```python
from build123d import *

# Parameters (mm, degrees)
SKETCH1_W           = 75
SKETCH1_H           = 90
BOSS_EXTRUDE1_DEPTH = 10
FILLET1_R           = 10
SKETCH3_W           = 75
SKETCH3_H           = 7.5
BOSS_EXTRUDE2_DEPTH = 60
FILLET2_R           = 7.5
SKETCH2_R           = 3
CUT_EXTRUDE1_DEPTH  = 10
CUT_EXTRUDE2_DEPTH  = 10
FILLET3_R           = 0.5
FILLET4_R           = 0.5


with BuildPart() as part:
    # Sketch1 → Boss-Extrude1 (new body)
    with BuildSketch(Plane.XY):
        Rectangle(SKETCH1_W, SKETCH1_H)
    extrude(amount=BOSS_EXTRUDE1_DEPTH)

    # Fillet1
    fillet1_edges = [part.edges().sort_by_distance(p)[0] for p in [
        (-37.5, 45, 5),
        (37.5, 45, 5),
    ]]
    fillet(fillet1_edges, radius=FILLET1_R)

    # Sketch3 → Boss-Extrude2 (add)
    with BuildSketch(Plane.XY.offset(10)):
        with Locations((0, -41.25)):
            Rectangle(SKETCH3_W, SKETCH3_H)
    extrude(amount=BOSS_EXTRUDE2_DEPTH)

    # Fillet2
    fillet2_edges = [part.edges().sort_by_distance(p)[0] for p in [
        (0, -37.5, 10),
    ]]
    fillet(fillet2_edges, radius=FILLET2_R)

    # Sketch2 → Cut-Extrude1 (cut)
    with BuildSketch(Plane.XY):
        with Locations(Location((23.999417703, 30, 0), (0, 0, 180))):
            Circle(SKETCH2_R)
        with Locations(Location((13.999417703, 30, 0), (0, 0, 180))):
            Circle(SKETCH2_R)
        with Locations(Location((3.999417703, 30, 0), (0, 0, 180))):
            Circle(SKETCH2_R)
        with Locations(Location((-6.000582297, 30, 0), (0, 0, 180))):
            Circle(SKETCH2_R)
        with Locations(Location((-16.000582297, 30, 0), (0, 0, 180))):
            Circle(SKETCH2_R)
        with Locations(Location((-26.000582297, 30, 0), (0, 0, 180))):
            Circle(SKETCH2_R)
        with Locations(Location((13.999417703, 15, 0), (0, 0, 180))):
            Circle(SKETCH2_R)
        with Locations(Location((3.999417703, 15, 0), (0, 0, 180))):
            Circle(SKETCH2_R)
        with Locations(Location((-6.000582297, 15, 0), (0, 0, 180))):
            Circle(SKETCH2_R)
        with Locations(Location((-16.000582297, 15, 0), (0, 0, 180))):
            Circle(SKETCH2_R)
        with Locations(Location((-26.000582297, 15, 0), (0, 0, 180))):
            Circle(SKETCH2_R)
        with Locations(Location((13.999417703, 0, 0), (0, 0, 180))):
            Circle(SKETCH2_R)
        with Locations(Location((3.999417703, 0, 0), (0, 0, 180))):
            Circle(SKETCH2_R)
        with Locations(Location((-6.000582297, 0, 0), (0, 0, 180))):
            Circle(SKETCH2_R)
        with Locations(Location((-16.000582297, 0, 0), (0, 0, 180))):
            Circle(SKETCH2_R)
        with Locations(Location((-26.000582297, 0, 0), (0, 0, 180))):
            Circle(SKETCH2_R)
        with Locations(Location((13.999417703, -15, 0), (0, 0, 180))):
            Circle(SKETCH2_R)
        with Locations(Location((3.999417703, -15, 0), (0, 0, 180))):
            Circle(SKETCH2_R)
        with Locations(Location((-6.000582297, -15, 0), (0, 0, 180))):
            Circle(SKETCH2_R)
        with Locations(Location((-16.000582297, -15, 0), (0, 0, 180))):
            Circle(SKETCH2_R)
        with Locations(Location((-26.000582297, -15, 0), (0, 0, 180))):
            Circle(SKETCH2_R)
        with Locations(Location((23.999417703, 15, 0), (0, 0, 180))):
            Circle(SKETCH2_R)
        with Locations(Location((23.999417703, 0, 0), (0, 0, 180))):
            Circle(SKETCH2_R)
        with Locations(Location((23.999417703, -15, 0), (0, 0, 180))):
            Circle(SKETCH2_R)
    extrude(amount=CUT_EXTRUDE1_DEPTH, mode=Mode.SUBTRACT)

    # Sketch4 → Cut-Extrude2 (cut)
    with BuildSketch(Plane(origin=(0, -37.5, 0), x_dir=(1, 0, 0), z_dir=(0, 1, 0))):
        with BuildLine():
            Line((-9.5, -26.25), (-9.5, -61.25))
            ThreePointArc((-9.5, -61.25), (-12.5, -64.25), (-15.5, -61.25))
            Line((-15.5, -61.25), (-15.5, -26.25))
            ThreePointArc((-15.5, -26.25), (-12.5, -23.25), (-9.5, -26.25))
        make_face()
        with BuildLine():
            Line((9.5, -26.25), (9.5, -61.25))
            ThreePointArc((9.5, -61.25), (12.5, -64.25), (15.5, -61.25))
            Line((15.5, -61.25), (15.5, -26.25))
            ThreePointArc((15.5, -26.25), (12.5, -23.25), (9.5, -26.25))
        make_face()
    extrude(amount=-CUT_EXTRUDE2_DEPTH, mode=Mode.SUBTRACT)

    # Fillet3
    fillet3_edges = [part.edges().sort_by_distance(p)[0] for p in [
        (0, -37.5, 70),
    ]]
    fillet(fillet3_edges, radius=FILLET3_R)

    # Fillet4
    fillet4_edges = [part.edges().sort_by_distance(p)[0] for p in [
        (0, 45, 10),
        (-37.5, 2.5, 10),
        (-34.571067812, 42.071067812, 10),
        (-37.5, -41.5, 70),
        (-37.5, -37.5, 43.5),
        (-37.5, -37.646446609, 69.853553391),
        (37.5, -37.5, 43.5),
        (37.5, -37.646446609, 69.853553391),
        (34.571067812, 42.071067812, 10),
        (37.5, -41.5, 70),
        (37.5, 2.5, 10),
        (-37.5, -35.303300859, 12.196699141),
        (37.5, -35.303300859, 12.196699141),
    ]]
    fillet(fillet4_edges, radius=FILLET4_R)


solid = part.part
```
Check sheet for the modelled part. Datum: model origin and axes. Units: mm. A direction names the side the tool comes from. Round coordinates to 2 decimals unless told otherwise and drop trailing zeros. Loops run counter-clockwise (first coordinate to the right, second up) from the corner with the lowest first, then second, coordinate; pieces in that order, holes last. Notation, with made-up numbers: (-2, -20) - (38, -20) arc R23 cw to (38, 6) - close; hole circle Ø1 at (43.25, 57). An arc over 180 degrees is marked (long way). Answer as a JSON object with one key per item and string values. Group by question number.
Q1. Sectioned sample at B-B, the plane x = 25. Enter the section's corners in (y, z), plus the area to 3 significant figures.
Q2. Scan lines: line 1 along Z through (x, y) = (-21.5, -20); line 2 along Y through (x, z) = (-16, 49); line 3 along Y through (x, z) = (-27.5, 4). Record each from-to range of solid material in increasing order. Write a range as [from, to].
Q3. Mould release check, pull along Z, two halves, no side actions. Record for faces 4 (the face through (-1, -41, 70)), 5 (the face through (-23, 30, 5)), 6 (the face through (-15.5, -41, 44)): released by +Z, released by -Z, zero draft, split by the parting line, or undercut.
Q4. Set-up check for faces 1 (the face through (4.65, -12.07, 4.93)), 2 (the face through (-1, 8, 10)), 3 (the face through (9.5, -41, 44)): record each of +Z, -Z, +X, -X, +Y, -Y from which the full face is reachable in a straight line by a thin tool's end or side.
Q5. Sectioned sample at C-C, the plane y = -15. Count the separate pieces of the cut face and the enclosed holes in it, plus the area to 3 significant figures.
Q6. Sectioned sample at A-A, the plane z = 41. Enter the section's corners in (x, y).
Q7. Gauge pin test, flat ends, axial feed: P1, Ø3.5, axis at x = -26, y = 30, coming from the +Z side; P2, Ø7, axis at x = -6, y = 30, coming from the +Z side; P3, Ø6, axis at x = 22, z = 48.5, coming from the +Y side. Record the tip position at first contact, or that the pin passes through.
Solution:
{
 "1": {"outline": "(-45, 0) - (-17.83, 0) - (-17.83, 10) - (-30, 10) arc R7.5 cw to (-37.5, 17.5) - (-37.5, 69.5) arc R0.5 ccw to (-38, 70) - (-45, 70) - close; (-12.17, 0) - (-2.83, 0) - (-2.83, 10) - (-12.17, 10) - close; (2.83, 0) - (12.17, 0) - (12.17, 10) - (2.83, 10) - close; (17.83, 0) - (27.17, 0) - (27.17, 10) - (17.83, 10) - close; (32.83, 0) - (45, 0) - (45, 9.5) arc R0.5 ccw to (44.5, 10) - (32.83, 10) - close", "area": "1,140 mm²"},
 "2": {"line 1": "z = [0, 10]", "line 2": "y = [-45, -37.5]", "line 3": "y = [-45, -17.6], [-12.4, -2.6], [2.6, 12.4], [17.6, 27.4], [32.6, 45]"},
 "3": {"face 4": "released by +Z", "face 5": "zero draft", "face 6": "undercut"},
 "4": {"face 1": "+Z, -Z", "face 2": "+Z, +X, -X, +Y", "face 3": "+Y, -Y"},
 "5": {"separate pieces": "7", "enclosed holes": "0", "area": "390 mm²"},
 "6": {"outline": "(-37.5, -45) - (-15.5, -45) - (-15.5, -37.5) - (-37, -37.5) arc R0.5 ccw to (-37.5, -38) - close; (-9.5, -45) - (9.5, -45) - (9.5, -37.5) - (-9.5, -37.5) - close; (15.5, -45) - (37.5, -45) - (37.5, -38) arc R0.5 ccw to (37, -37.5) - (15.5, -37.5) - close"},
 "7": {"P1": "passes through", "P2": "stops at z = 10", "P3": "stops at y = -37.5"}
}
